from build123d import *

# Parameters (mm, degrees)
F1_DEPTH      = 5
F0_R          = 2
F2_DEPTH      = 10
F2_DEPTH_BACK = 5
F3_DEPTH      = 10


with BuildPart() as f1:
    # F0 (on Front) → F1 (new body)
    with BuildSketch(Plane.XZ):
        Polygon((0, 43), (0, 0), (43, 0), (43, 10), (10, 10), (10, 43), align=None)
    extrude(amount=-F1_DEPTH)

    # F0 (on Front) → F2 (join, two sides)
    with BuildSketch(Plane.XZ) as f2_sk:
        with BuildLine():
            Line((10, 10), (43, 10))
            Line((43, 10), (43, 14))
            ThreePointArc((43, 14), (34.506097, 34.506097), (14, 43))
            Line((14, 43), (10, 43))
            Line((10, 43), (10, 10))
        make_face()
        with Locations((14, 14)):
            Circle(F0_R, mode=Mode.SUBTRACT)
    extrude(amount=F2_DEPTH)
    extrude(f2_sk.sketch, amount=-F2_DEPTH_BACK)

    # F0 (on Front) → F3 (join)
    with BuildSketch(Plane.XZ):
        with BuildLine():
            Line((43, 14), (43, 10))
            Line((43, 10), (53, 10))
            Line((53, 10), (53, 14))
            ThreePointArc((53, 14), (41.577164, 41.577164), (14, 53))
            Line((14, 53), (10, 53))
            Line((10, 53), (10, 43))
            Line((10, 43), (14, 43))
            ThreePointArc((14, 43), (34.506097, 34.506097), (43, 14))
        make_face()
    extrude(amount=F3_DEPTH)


solid = f1.part
For this review, take the finished solid that the model builds, in its own axes (mm). A direction names the side the tool comes from. Round coordinates to 2 decimals unless told otherwise and drop trailing zeros. Loops run counter-clockwise (first coordinate to the right, second up) from the corner with the lowest first, then second, coordinate; pieces in that order, holes last. Notation, with made-up numbers: (41, 89.5) - (54, 89.5) arc R22 ccw to (54, 95.5) - close; hole circle Ø4 at (66.25, -2.75). An arc over 180 degrees is marked (long way). Answer as CSV lines item,"result".
(1) Tool access review of faces 5 (the face through (21, 5, 22)), 6 (the face through (7, 2, 43)), 7 (the face through (41.88, -4.93, 41.27)), 8 (the face through (43, 2, 7)), 9 (the face through (35, 0, 35)): name each direction out of +Z, -Z, +X, -X, +Y, -Y from which nothing blocks a thin tool from reaching the whole face with its end or side.
Checked values:
face 5,"+Z, -Z, +X, -X, +Y"
face 6,"+Z, +X, -X, +Y"
face 7,"+Z, +X, +Y, -Y"
face 8,"+Z, -Z, +X, +Y"
face 9,"+Z, +X, +Y"
(2) Mouldability with a two-part tool opening along Z and no side actions: class faces 1 (the face through (35, 2, 34)), 2 (the face through (10, -5, 32)), 3 (the face through (12.526, -2.395, 15.352)), 4 (the face through (31, -5, 10)) as +Z half, -Z half, draft (parallel to the pull), parting line (faces both ways), or undercut.
Checked values:
face 1,"+Z half"
face 2,"draft"
face 3,"undercut"
face 4,"-Z half"
(3) Wall thickness on line 1 (Z direction, x = 14, y = -2); line 2 (Y direction, x = 13, z = 7); line 3 (Y direction, x = 38.5, z = 41.5): over which ranges is each line inside the solid? List them lowest first.
Checked values:
line 1,"z = 10 to 12, 16 to 53"
line 2,"y = 0 to 5"
line 3,"y = -10 to 0"
(4) Consider section D-D on y = 2.5. Give the boundary of the cut face in (x, z), then the cut area to 3 significant figures.
Checked values:
outline,"(0, 0) - (43, 0) - (43, 14) arc R29 ccw to (14, 43) - (0, 43) - close; hole circle Ø4 at (14, 14)"
area,"1,660 mm2"
(5) Consider section A-A on y = -1.75. Give the boundary of the cut face in (x, z), then the cut area to 3 significant figures.
Checked values:
outline,"(10, 10) - (53, 10) - (53, 14) arc R39 ccw to (14, 53) - (10, 53) - close; hole circle Ø4 at (14, 14)"
area,"1,510 mm2"
(6) Consider section B-B on z = 37. Give the boundary of the cut face in (x, y).
Checked values:
outline,"(0, 0) - (10, 0) - (10, -10) - (45.5, -10) - (45.5, 0) - (31.66, 0) - (31.66, 5) - (0, 5) - close"
(7) Consider section C-C on x = 18. Give the boundary of the cut face in (y, z).
Checked values:
outline,"(-10, 10) - (0, 10) - (0, 0) - (5, 0) - (5, 42.72) - (0, 42.72) - (0, 52.79) - (-10, 52.79) - close"
(8) Insertion check: P1, Ø3, axis at x = 31.5, y = -3.5, coming from the -Z side; P2, Ø2.5, axis at x = 3.5, y = 2.5, coming from the +Z side. Each pin has a flat end and moves straight along its axis. Give the tip position at first contact, or say it passes through.
Checked values:
P1,"stops at z = 10"
P2,"stops at z = 43"
